Check sheet for the drawn part. Datum: minimum x, y, z corner. Units: mm. A direction names the side the tool comes from. Give positions to 0.01 mm unless a question says otherwise; leave off trailing zeros. Loops run counter-clockwise (first coordinate to the right, second up) from the corner with the lowest first, then second, coordinate; pieces in that order, holes last. Notation, with made-up numbers: (60, -29.5) -> (112, -29.5) arc R27 cw to (112, -9.5) -> close; hole circle Ø9 at (-20, -4.5). An arc over 180 degrees is marked (long way). One line per question, with ' | ' between items.
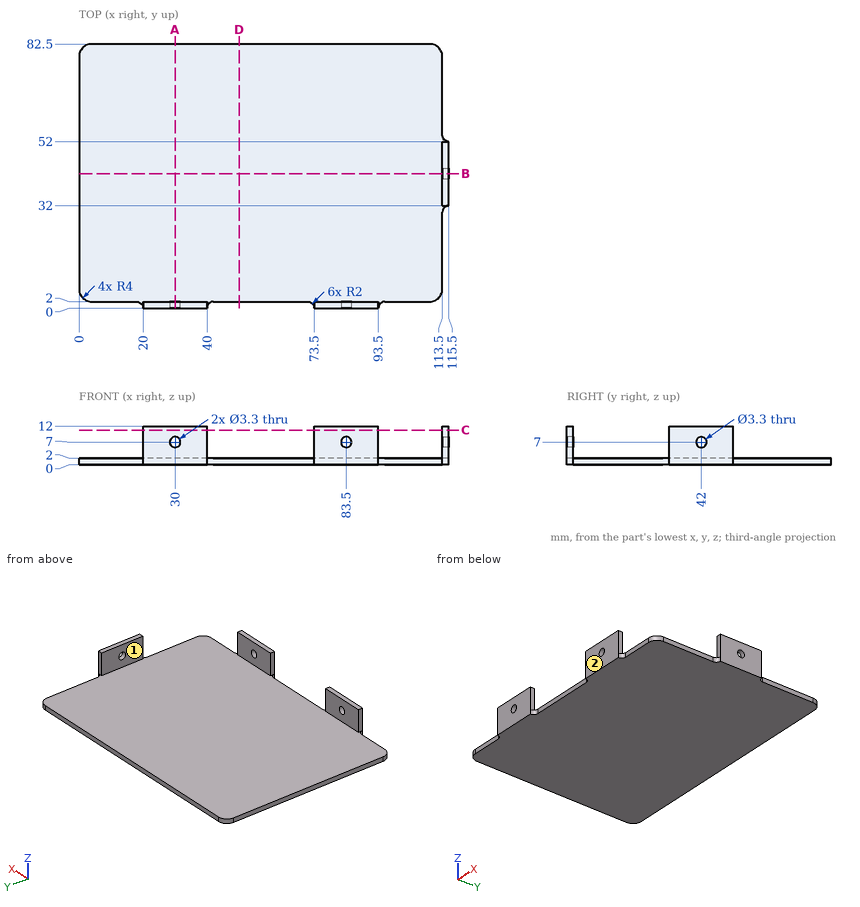
Item 1: Sectioned sample at B-B (y = 42). Record the cut outline in (x, z), plus the area to 3 significant figures.
Result:
outline: (0, 0) -> (115.5, 0) -> (115.5, 5.35) -> (113.5, 5.35) -> (113.5, 2) -> (0, 2) -> close; (113.5, 8.65) -> (115.5, 8.65) -> (115.5, 12) -> (113.5, 12) -> close | area: 244 mm2
Item 2: Scan lines: probe 1 along Z at (x, y) = (30, 1); probe 2 along Y at (x, z) = (114.9, 7); probe 3 along Z at (x, y) = (27, 16). Record each from-to range of solid material in increasing order.
Result:
probe 1: 0 to 5.35, 8.65 to 12 | probe 2: 32 to 40.35, 43.65 to 52 | probe 3: 0 to 2
Item 3: Sectioned sample at A-A (x = 30). Record the cut outline in (y, z).
Result:
outline: (0, 0) -> (82.5, 0) -> (82.5, 2) -> (2, 2) -> (2, 5.35) -> (0, 5.35) -> close; (0, 8.65) -> (2, 8.65) -> (2, 12) -> (0, 12) -> close
Item 4: Sectioned sample at C-C (z = 10.75). Record the cut outline in (x, y), plus the area to 3 significant figures.
Result:
outline: (20, 0) -> (40, 0) -> (40, 2) -> (20, 2) -> close; (73.5, 0) -> (93.5, 0) -> (93.5, 2) -> (73.5, 2) -> close; (113.5, 32) -> (115.5, 32) -> (115.5, 52) -> (113.5, 52) -> close | area: 120 mm2
Item 5: Set-up check for the marked faces 1 and 2: record each of +Z, -Z, +X, -X, +Y, -Y from which the full face is reachable in a straight line by a thin tool's end or side.
Result:
face 1: +Z, -X, +Y, -Y | face 2: +Z, -Z, +X, -X, -Y
Item 6: Depth check by flat-ended pin: pin 1 Ø0.6 at (y, z) = (1, 8) entering from -X; pin 2 Ø0.6 at (y, z) = (16.5, 1) entering from +X; pin 3 Ø10 at (x, y) = (31.5, 51) entering from +Z. Enter the tip coordinate at first touch or a pass-through.
Result:
pin 1: x = 20 | pin 2: x = 113.5 | pin 3: z = 2
Item 7: Sectioned sample at D-D (x = 50). Record the cut outline in (y, z).
Result:
outline: (2, 0) -> (82.5, 0) -> (82.5, 2) -> (2, 2) -> close
